```python
from build123d import *

# Parameters (mm, degrees)
CHAFL_N2_SIZE          = 1.5
CHAFL_N3_SIZE          = 1.5
CROQUIS2_R             = 2.5
CROQUIS2_W             = 5
CROQUIS2_H             = 0.5
CROQUIS5_R             = 25
CORTAR_EXTRUIR5_DEPTH  = 300
CROQUIS3_W             = 50
CROQUIS3_H             = 50
CORTAR_EXTRUIR9_DEPTH  = 6.5
CROQUIS7_R             = 5
CORTAR_EXTRUIR12_DEPTH = 46.5


with BuildPart() as part:
    # Croquis1 → Revolución1 (revolve)
    with BuildSketch(Plane(origin=(0, 0, 0), x_dir=(1, 0, 0), z_dir=(0, 1, 0)), mode=Mode.PRIVATE) as revoluci_n1_sk:
        Polygon((-25, 37.5), (25, 37.5), (25, 35), (125, 35), (125, 0), (-125, 0), (-125, 35), (-25, 35), align=None)
    revolve(revoluci_n1_sk.sketch.rotate(Axis((-200, 0, 0), (1, 0, 0)), 180), axis=Axis((-200, 0, 0), (1, 0, 0)))

    # Chaflán2
    chafl_n2_edges = [part.edges().sort_by_distance(p)[0] for p in [
        (-125, 0, -35),
    ]]
    chamfer(chafl_n2_edges, length=CHAFL_N2_SIZE)

    # Chaflán3
    chafl_n3_edges = [part.edges().sort_by_distance(p)[0] for p in [
        (125, 0, -35),
    ]]
    chamfer(chafl_n3_edges, length=CHAFL_N3_SIZE)

    # Croquis2 → Cortar-Revolución1 (revolve, cut)
    with BuildSketch(Plane.XY, mode=Mode.PRIVATE) as cortar_revoluci_n1_sk:
        with Locations((0, 37.5)):
            Circle(CROQUIS2_R)
        with Locations((-27.5, 34.75)):
            Rectangle(CROQUIS2_W, CROQUIS2_H)
        with Locations((27.5, 34.75)):
            Rectangle(CROQUIS2_W, CROQUIS2_H)
    revolve(cortar_revoluci_n1_sk.sketch.rotate(Axis((-200, 0, 0), (1, 0, 0)), 90), axis=Axis((-200, 0, 0), (1, 0, 0)), mode=Mode.SUBTRACT)

    # Croquis5 → Cortar-Extruir5 (cut)
    with BuildSketch(Plane(origin=(125, 0, 0), x_dir=(0, 0, -1), z_dir=(1, 0, 0))):
        Circle(CROQUIS5_R)
    extrude(amount=-CORTAR_EXTRUIR5_DEPTH, mode=Mode.SUBTRACT)

    # Croquis3 → Cortar-Extruir9 (cut)
    with BuildSketch(Plane.XY.offset(35)):
        with Locations((91.5, 0)):
            Rectangle(CROQUIS3_W, CROQUIS3_H)
        with Locations((-91.5, 0)):
            Rectangle(CROQUIS3_W, CROQUIS3_H)
    extrude(amount=-CORTAR_EXTRUIR9_DEPTH, mode=Mode.SUBTRACT)

    # Croquis7 → Cortar-Extruir12 (cut)
    with BuildSketch(Plane.XY.offset(28.5)):
        with Locations((-105.5, 0)):
            Circle(CROQUIS7_R)
        with Locations((105.5, 0)):
            Circle(CROQUIS7_R)
    extrude(amount=-CORTAR_EXTRUIR12_DEPTH, mode=Mode.SUBTRACT)


solid = part.part
```
The model under review builds one solid part; all positions refer to its coordinate system, in mm. A direction names the side the tool comes from. Round coordinates to 2 decimals unless told otherwise and drop trailing zeros. Order: outer loops, then holes, each group sorted by start corner. A loop starts at its lowest first (then second) coordinate and runs counter-clockwise, first axis right, second up. Notation, with made-up numbers: (89.25, 80) -> (144.25, 80) arc R14 ccw to (144.25, 100) -> close; hole circle Ø5 at (69, -19.5). An arc over 180 degrees is marked (long way). Use a Markdown table: item, result.
Q1. Mouldability with a two-part tool opening along Y and no side actions: class faces 1 (the cylindrical face through (27.535, -1.517, -34.467)), 2 (the flat face through (30, 26, -23)), 3 (the cylindrical face through (110.119, -1.915, 26.525)) as +Y half, -Y half, draft (parallel to the pull), parting line (faces both ways), or undercut.
Values:
| item | result |
|---|---|
| face 1 | parting line |
| face 2 | draft |
| face 3 | undercut |
Q2. We need section C-C on y = 0. State how many separate pieces and enclosed holes the cut face has, then the cut area to 3 significant figures.
Values:
| item | result |
|---|---|
| separate pieces | 4 |
| enclosed holes | 0 |
| area | 4,500 mm^2 |
Q3. Tool access review of faces 4 (the flat face through (-66.5, 0, 31)), 5 (the cylindrical face through (-100.881, -1.915, 26.525)), 6 (the flat face through (-30, 26, -23)), 7 (the cylindrical face through (-76.096, -1.539, -34.966)): name each direction out of +Z, -Z, +X, -X, +Y, -Y from which nothing blocks a thin tool from reaching the whole face with its end or side.
Values:
| item | result |
|---|---|
| face 4 | +Z, +Y, -Y |
| face 5 | +Z |
| face 6 | none |
| face 7 | -X |
Q4. We need section B-B on x = 105.5. Write out the cut boundary in (y, z), then the cut area to 3 significant figures.
Values:
| item | result |
|---|---|
| outline | (-20.32, 28.5) arc R35 ccw (long way) to (20.32, 28.5) -> (5, 28.5) -> (5, 24.49) arc R25 cw (long way) to (-5, 24.49) -> (-5, 28.5) -> close |
| area | 1,670 mm^2 |
Q5. We need section D-D on x = -56.5. Write out the cut boundary in (y, z), then the cut area to 3 significant figures.
Values:
| item | result |
|---|---|
| outline | circle Ø70 at (0, 0); hole circle Ø50 at (0, 0) |
| area | 1,880 mm^2 |
Q6. Clearance check with flat-ended pins moving along their axes: P1, Ø12, axis at x = 89.5, y = -15, coming from the +Z side; P2, Ø6, axis at x = -65, y = -10, coming from the -Z side; P3, Ø1.5, axis at x = -33, z = 4, coming from the -Y side. State where each tip first meets the part, or that it passes through.
Values:
| item | result |
|---|---|
| P1 | stops at z = 28.5 |
| P2 | stops at z = -34.29 |
| P3 | stops at y = -34.85 |
Q7. For line 1 (Y direction, x = -69.5, z = -1); line 2 (Z direction, x = 69, y = 0); line 3 (X direction, y = -31, z = -20.5), list the stretches that pass through material, from the lowest coordinate up.
Values:
| item | result |
|---|---|
| line 1 | y = -34.99 to -24.98, 24.98 to 34.99 |
| line 2 | z = -35 to -25, 25 to 28.5 |
| line 3 | x = -25 to -2.48, 2.48 to 25 |
